Check sheet for the modelled part. Datum: model origin and axes. Units: mm. Give positions to 0.01 mm unless a question says otherwise; leave off trailing zeros. Write each loop counter-clockwise with the first axis right and the second up, starting at its lowest first coordinate (ties: lowest second). Pieces come first, ordered by that corner, then holes. Notation, with made-up numbers: (-31.75, 29.5) -> (-5.75, 29.5) arc R15 cw to (-5.75, 38.5) -> close; hole circle Ø4 at (46, -39.75). An arc over 180 degrees is marked (long way). Use a Markdown table: item, result. Add a question column.
1. Cross-section at A-A (y = 51.5). Enter the section's corners in (x, z), then the cut area to 3 significant figures.
2. Scan lines: probe 1 along Y at (x, z) = (0, 2.2) (3 decimals); probe 2 along X at (y, z) = (46, 1.8); probe 3 along Y at (x, z) = (4.5, 0.8). Record each from-to range of solid material in increasing order. Write a range as [from, to].
3. Cross-section at C-C (x = 7.5). Enter the section's corners in (y, z).
4. Gauge pin test, flat ends, axial feed: P1, Ø2.5, axis at x = -20.35, y = -11.75, coming from the -Z side; P2, Ø2, axis at y = 68, z = 2.5, coming from the +X side; P3, Ø1.2, axis at x = 15.5, z = 1, coming from the -Y side. Record the tip position at first contact, or that the pin passes through.
5. Cross-section at D-D (y = 11.75). Enter the section's corners in (x, z), then the cut area to 3 significant figures.
6. Cross-section at B-B (x = 0). Enter the section's corners in (y, z) (3 decimals), then the cut area to 3 significant figures.
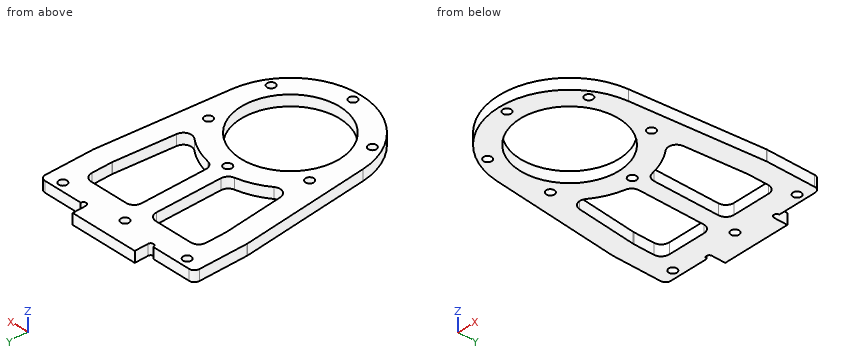
from build123d import *

# Parameters (mm, degrees)
SKETCH_1_R          = 18.5
EXTRUDE_1_DEPTH     = 4
CUT_EXTRUDE_1_DEPTH = 10
SKETCH_3_R          = 1.525
CUT_EXTRUDE_2_DEPTH = 22
SKETCH_4_R          = 1.525
CUT_EXTRUDE_3_DEPTH = 22
FILLET_1_R          = 2
SKETCH_5_W          = 25
SKETCH_5_H          = 5
EXTRUDE_2_DEPTH     = 4
SKETCH_6_R          = 1.05
CUT_EXTRUDE_4_DEPTH = 4
CUT_EXTRUDE_5_DEPTH = 52
FILLET_3_R          = 3


with BuildPart() as part:
    # 草图1 → 凸台-拉伸1 (new body)
    with BuildSketch(Plane.XY):
        with BuildLine():
            Line((-31, 0), (-31, 65))
            Line((-31, 65), (31, 65))
            Line((31, 65), (31, 0))
            ThreePointArc((31, 0), (0, -31), (-31, 0))
        make_face()
        Circle(SKETCH_1_R, mode=Mode.SUBTRACT)
    extrude(amount=EXTRUDE_1_DEPTH)

    # 草图2 → 切除-拉伸1 (cut)
    with BuildSketch(Plane.XY.offset(4)):
        with BuildLine():
            Line((-26.375636933, -2.564327665), (-31, 45))
            Line((-31, 45), (-31, -32))
            Line((-31, -32), (31, -32))
            Line((31, -32), (31, 45))
            Line((31, 45), (26.375636933, -2.564327665))
            ThreePointArc((26.375636933, -2.564327665), (0, -26.5), (-26.375636933, -2.564327665))
        make_face()
    extrude(amount=-CUT_EXTRUDE_1_DEPTH, mode=Mode.SUBTRACT)

    # 草图3 → 切除-拉伸2 (cut)
    with BuildSketch(Plane.XY.offset(4)):
        with Locations((0, 23.5)):
            Circle(SKETCH_3_R)
        with Locations((20.351596989, 11.75)):
            Circle(SKETCH_3_R)
        with Locations((20.351596989, -11.75)):
            Circle(SKETCH_3_R)
        with Locations((0, -23.5)):
            Circle(SKETCH_3_R)
        with Locations((-20.351596989, -11.75)):
            Circle(SKETCH_3_R)
        with Locations((-20.351596989, 11.75)):
            Circle(SKETCH_3_R)
    extrude(amount=-CUT_EXTRUDE_2_DEPTH, mode=Mode.SUBTRACT)

    # 草图4 → 切除-拉伸3 (cut)
    with BuildSketch(Plane.XY.offset(4)):
        with Locations((25, 62)):
            Circle(SKETCH_4_R)
        with Locations((0, 62)):
            Circle(SKETCH_4_R)
        with Locations((-25, 62)):
            Circle(SKETCH_4_R)
    extrude(amount=-CUT_EXTRUDE_3_DEPTH, mode=Mode.SUBTRACT)

    # 圆角1
    # the kernel refuses this fillet: 2 mm, written as the material it takes off along each edge
    with BuildSketch(Plane(origin=(-31, 45, 4.242486693), x_dir=(0, 1, 0), z_dir=(0, 0, -1)), Plane(origin=(31, 45, 4.242486693), x_dir=(-0.09676708169889991, -0.9953070540790306, 0), z_dir=(0, 0, -1))) as fillet_1_piece_1:
        with BuildLine():
            CenterArc((FILLET_1_R * 0.048497338543, FILLET_1_R), FILLET_1_R, 264.446965205, 5.553034795)
            Line((-FILLET_1_R * 0.0482697431559, FILLET_1_R * 0.00469294592097), (0, 0))
            Line((0, 0), (FILLET_1_R * 0.048497338543, 0))
        make_face()
    extrude(amount=4.484973385, mode=Mode.SUBTRACT)
    with BuildSketch(Plane(origin=(-31, 65, -5), x_dir=(0, -1, 0), z_dir=(0, 0, 1)), Plane(origin=(31, 65, -5), x_dir=(-1, 0, 0), z_dir=(0, 0, 1))) as fillet_1_piece_2:
        with BuildLine():
            CenterArc((FILLET_1_R, FILLET_1_R), FILLET_1_R, 180, 90)
            Line((0, FILLET_1_R), (0, 0))
            Line((0, 0), (FILLET_1_R, 0))
        make_face()
    extrude(amount=14, mode=Mode.SUBTRACT)

    # 草图5 → 凸台-拉伸2 (add)
    with BuildSketch(Plane.XY.offset(4)):
        with Locations((0, 67.5)):
            Rectangle(SKETCH_5_W, SKETCH_5_H)
    extrude(amount=-EXTRUDE_2_DEPTH)

    # 草图6 → 切除-拉伸4 (cut)
    with BuildSketch(Plane(origin=(0, 0, 0), x_dir=(-1, 0, 0), z_dir=(0, 0, -1))):
        with Locations((13.55, 65)):
            Circle(SKETCH_6_R)
        with Locations((-13.55, 65)):
            Circle(SKETCH_6_R)
    extrude(amount=-CUT_EXTRUDE_4_DEPTH, mode=Mode.SUBTRACT)

    # 草图7 → 切除-拉伸5 (cut)
    with BuildSketch(Plane.XY.offset(4)):
        with BuildLine():
            Line((-3, 26.329641091), (-3, 56))
            Line((-3, 56), (-23, 56))
            Line((-23, 56), (-23, 45.387978708))
            Line((-23, 45.387978708), (-20.249206785, 17.094432561))
            ThreePointArc((-20.249206785, 17.094432561), (-12.508144274, 23.362284281), (-3, 26.329641091))
        make_face()
        with BuildLine():
            Line((3, 56), (3, 26.329641091))
            ThreePointArc((3, 26.329641091), (12.508144274, 23.362284281), (20.249206785, 17.094432561))
            Line((20.249206785, 17.094432561), (23, 45.387978708))
            Line((23, 45.387978708), (23, 56))
            Line((23, 56), (3, 56))
        make_face()
    extrude(amount=-CUT_EXTRUDE_5_DEPTH, mode=Mode.SUBTRACT)

    # 圆角3
    # the kernel refuses this fillet: 3 mm, written as the material it adds along each edge
    with BuildSketch(Plane(origin=(-3, 26.329641091, 4), x_dir=(0, 1, 0), z_dir=(0, 0, -1))) as fillet_3_piece_1:
        with BuildLine():
            CenterArc((2.553745137, -3), FILLET_3_R, 90, 78.264742526)
            ThreePointArc((-0.383548378, -2.389830508), (-0.164475151, -1.199296528), (0, 0))
            Line((0, 0), (2.553745137, 0))
        make_face()
    extrude(amount=4)
    with BuildSketch(Plane(origin=(-20.249206785, 17.094432561, 4), x_dir=(0.7249016624604615, 0.6888523642712269, 0), z_dir=(0, 0, -1))) as fillet_3_piece_2:
        with BuildLine():
            CenterArc((6.134944493, -2.981943006), FILLET_3_R, 96.289524431, 121.69677285)
            Line((3.770470579, -4.828362003), (0, 0))
            ThreePointArc((0, 0), (2.903143376, -0.159503449), (5.806286752, 0))
        make_face()
    extrude(amount=4)
    with BuildSketch(Plane(origin=(-23, 45.387978708, 4), x_dir=(0.09676708169889287, -0.9953070540790314, 0), z_dir=(0, 0, -1)), Plane(origin=(23, 45.387978708, 4), x_dir=(0, 1, 0), z_dir=(0, 0, -1))) as fillet_3_piece_3:
        with BuildLine():
            CenterArc((FILLET_3_R * 0.048497338543, -FILLET_3_R), FILLET_3_R, 90, 5.553034795)
            Line((-FILLET_3_R * 0.0482697431559, -FILLET_3_R * 0.00469294592097), (0, 0))
            Line((0, 0), (FILLET_3_R * 0.048497338543, 0))
        make_face()
    extrude(amount=4)
    with BuildSketch(Plane(origin=(-23, 56, 4), x_dir=(0, -1, 0), z_dir=(0, 0, -1)), Plane(origin=(3, 56, 4), x_dir=(0, -1, 0), z_dir=(0, 0, -1)), Plane(origin=(23, 56, 4), x_dir=(-1, 0, 0), z_dir=(0, 0, -1))) as fillet_3_piece_4:
        with BuildLine():
            CenterArc((FILLET_3_R, -FILLET_3_R), FILLET_3_R, 90, 90)
            Line((0, -FILLET_3_R), (0, 0))
            Line((0, 0), (FILLET_3_R, 0))
        make_face()
    extrude(amount=4)
    with BuildSketch(Plane(origin=(-3, 56, 4), x_dir=(0, -1, 0), z_dir=(0, 0, -1))) as fillet_3_piece_5:
        with BuildLine():
            CenterArc((FILLET_3_R, FILLET_3_R), FILLET_3_R, 180, 90)
            Line((0, FILLET_3_R), (0, 0))
            Line((0, 0), (FILLET_3_R, 0))
        make_face()
    extrude(amount=4)
    with BuildSketch(Plane(origin=(20.249206785, 17.094432561, 4), x_dir=(0.09676708169888887, 0.9953070540790317, 0), z_dir=(0, 0, -1))) as fillet_3_piece_6:
        with BuildLine():
            CenterArc((6.126134835, -3), FILLET_3_R, 90, 121.69677285)
            ThreePointArc((3.57361272, -4.576271186), (1.912520275, -2.189965527), (0, 0))
            Line((0, 0), (6.126134835, 0))
        make_face()
    extrude(amount=4)
    with BuildSketch(Plane(origin=(3, 26.329641091, 4), x_dir=(0, 1, 0), z_dir=(0, 0, -1))) as fillet_3_piece_7:
        with BuildLine():
            CenterArc((2.553745137, 3), FILLET_3_R, 191.735257474, 78.264742526)
            ThreePointArc((-0.383548378, 2.389830508), (-0.164475151, 1.199296528), (0, 0))
            Line((0, 0), (2.553745137, 0))
        make_face()
    extrude(amount=4)


solid = part.part
Worked answers:
| question | item | result |
|---|---|---|
| 1 | outline | (-31, 0) -> (-23, 0) -> (-23, 4) -> (-31, 4) -> close; (-3, 0) -> (3, 0) -> (3, 4) -> (-3, 4) -> close; (23, 0) -> (31, 0) -> (31, 4) -> (23, 4) -> close |
| 1 | area | 88.0 mm² |
| 2 | probe 1 | y = [-26.5, -25.025], [-21.975, -18.5], [18.5, 21.975], [25.025, 60.475], [63.525, 70] |
| 2 | probe 2 | x = [-31, -23], [-3, 3], [23, 31] |
| 2 | probe 3 | y = [-26.12, -17.94], [17.94, 26.29], [55.6, 70] |
| 3 | outline | (-25.42, 0) -> (-16.91, 0) -> (-16.91, 4) -> (-25.42, 4) -> close; (16.91, 0) -> (25.42, 0) -> (25.42, 4) -> (16.91, 4) -> close; (56, 0) -> (70, 0) -> (70, 4) -> (56, 4) -> close |
| 4 | P1 | passes through |
| 4 | P2 | stops at x = 12.5 |
| 4 | P3 | stops at y = -21.91 |
| 5 | outline | (-27.77, 0) -> (-21.88, 0) -> (-21.88, 4) -> (-27.77, 4) -> close; (-18.83, 0) -> (-14.29, 0) -> (-14.29, 4) -> (-18.83, 4) -> close; (14.29, 0) -> (18.83, 0) -> (18.83, 4) -> (14.29, 4) -> close; (21.88, 0) -> (27.77, 0) -> (27.77, 4) -> (21.88, 4) -> close |
| 5 | area | 83.4 mm² |
| 6 | outline | (-26.5, 0) -> (-25.025, 0) -> (-25.025, 4) -> (-26.5, 4) -> close; (-21.975, 0) -> (-18.5, 0) -> (-18.5, 4) -> (-21.975, 4) -> close; (18.5, 0) -> (21.975, 0) -> (21.975, 4) -> (18.5, 4) -> close; (25.025, 0) -> (60.475, 0) -> (60.475, 4) -> (25.025, 4) -> close; (63.525, 0) -> (70, 0) -> (70, 4) -> (63.525, 4) -> close |
| 6 | area | 201 mm² |
